Geometry check sheet. Reference: drawing and pictorial views, mm from the part's lowest x, y, z. A direction names the side the tool comes from. Round coordinates to 2 decimals unless told otherwise and drop trailing zeros. Order: outer loops, then holes, each group sorted by start corner. A loop starts at its lowest first (then second) coordinate and runs counter-clockwise, first axis right, second up.
(1) Depth check by flat-ended pin: pin 1 (3 mm diameter, centred on x = 14, z = 6.5, fed in from +Y); pin 2 (4 mm diameter, centred on y = 18.5, z = 4.5, fed in from -X); pin 3 (1 mm diameter, centred on y = 25, z = 1.5, fed in from +X); pin 4 (12 mm diameter, centred on x = 7, y = 6.5, fed in from -Z). Enter the tip coordinate at first touch or a pass-through.
(2) Sectioned sample at C-C, the plane y = 9.5. Enter the section's corners in (x, z).
(3) Tool access check on the marked faces 4 and 5. Record the directions out of +Z, -Z, +X, -X, +Y, -Y that give a thin tool (end or side, any length) a straight path to the whole face; none if there is none.
(4) Sectioned sample at B-B, the plane x = 12. Enter the section's corners in (y, z).
(5) Thickness scan on probe 1 along X at (y, z) = (4.5, 5.5); probe 2 along Z at (x, y) = (13.5, 19); probe 3 along Y at (x, z) = (4.5, 1.75). Record the ranges inside material, lowest first.
(6) Mould release check, pull along X, two halves, no side actions. Record for the marked faces 1, 2 and 3: released by +X, released by -X, zero draft, split by the parting line, or undercut.
(7) Sectioned sample at A-A, the plane z = 3.75. Enter the section's corners in (x, y).
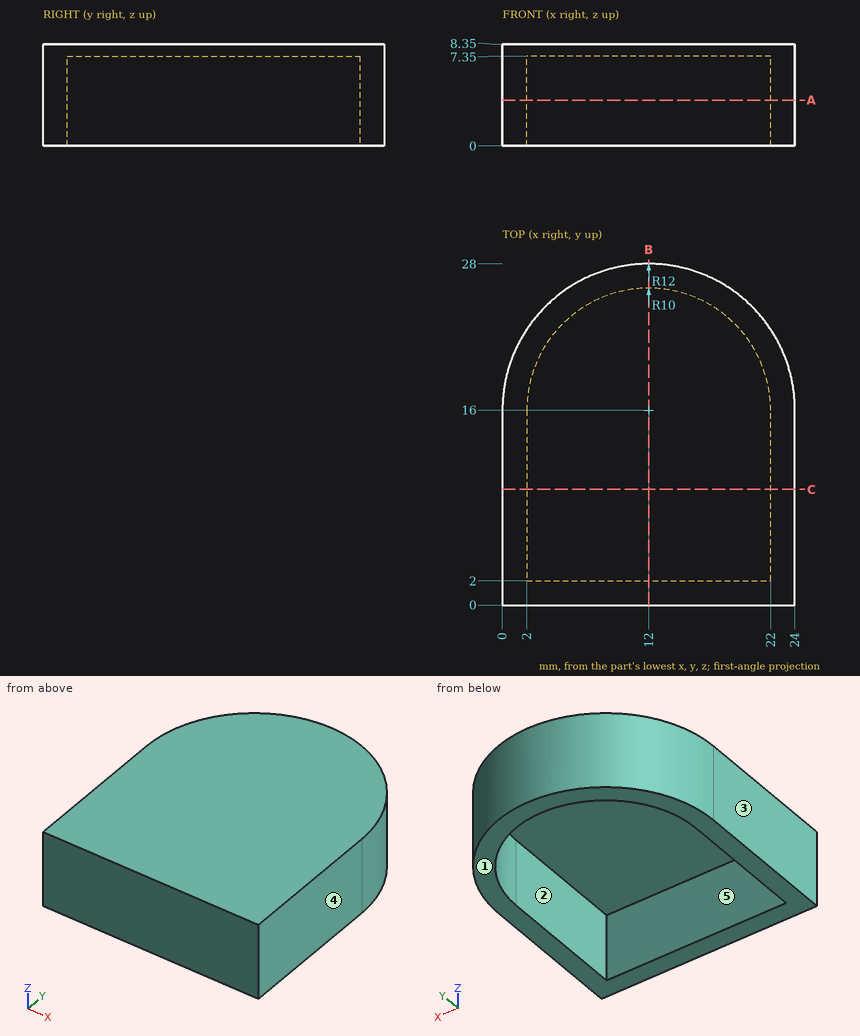
Derived:
1. pin 1: stops at y = 27.99
1. pin 2: stops at x = 0.01
1. pin 3: stops at x = 20.47
1. pin 4: stops at z = 0
2. outline: (0, 0) - (2, 0) - (2, 7.35) - (22, 7.35) - (22, 0) - (24, 0) - (24, 8.35) - (0, 8.35) - close
3. face 4: +Z, -Z, +X, +Y, -Y
3. face 5: -Z
4. outline: (0, 0) - (2, 0) - (2, 7.35) - (26, 7.35) - (26, 0) - (28, 0) - (28, 8.35) - (0, 8.35) - close
5. probe 1: x = 0 to 2, 22 to 24
5. probe 2: z = 7.35 to 8.35
5. probe 3: y = 0 to 2, 22.61 to 25.37
6. face 1: zero draft
6. face 2: undercut
6. face 3: released by -X
7. outline: (0, 0) - (24, 0) - (24, 16) arc R12 ccw to (0, 16) - close; hole (2, 2) - (22, 2) - (22, 16) arc R10 ccw to (2, 16) - close
